Could you check a few things on this model? Use its own coordinates, in mm. Face numbers are marked on the shaded views. A direction names the side the tool comes from. Coordinates: 2 decimals unless noted, no trailing zeros. Order: outer loops, then holes, each group sorted by start corner. A loop starts at its lowest first (then second) coordinate and runs counter-clockwise, first axis right, second up. Notation, with made-up numbers: (63.25, -21.5) - (113.25, -21.5) arc R26 cw to (113.25, -3.5) - close; hole circle Ø7 at (11, -20). An arc over 180 degrees is marked (long way). One line per item, written item: value. Start each with the question number.
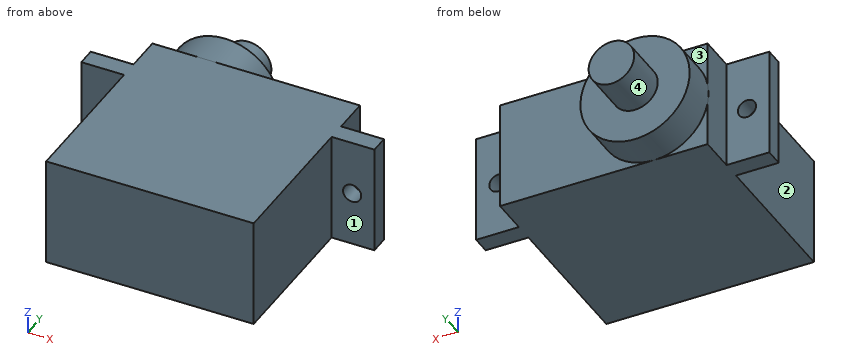
from build123d import *

# Parameters (mm, degrees)
SKETCH1_W           = 22.8
SKETCH1_H           = 12
BOSS_EXTRUDE1_DEPTH = 22.5
SKETCH2_W           = 12
SKETCH2_H           = 2
BOSS_EXTRUDE2_DEPTH = 4.7
SKETCH3_R           = 6
BOSS_EXTRUDE3_DEPTH = 4
SKETCH4_R           = 2.5
BOSS_EXTRUDE4_DEPTH = 5
SKETCH5_R           = 1
CUT_EXTRUDE1_DEPTH  = 5


with BuildPart() as part:
    # Sketch1 → Boss-Extrude1 (new body)
    with BuildSketch(Plane(origin=(0, 0, 0), x_dir=(1, 0, 0), z_dir=(0, 1, 0))):
        Rectangle(SKETCH1_W, SKETCH1_H)
    extrude(amount=BOSS_EXTRUDE1_DEPTH)

    # Sketch2 → Boss-Extrude2 (add)
    with BuildSketch(Plane(origin=(11.4, 0, 0), x_dir=(0, 0, -1), z_dir=(1, 0, 0))):
        with Locations((0, 17.5)):
            Rectangle(SKETCH2_W, SKETCH2_H)
    boss_extrude2 = extrude(amount=BOSS_EXTRUDE2_DEPTH)

    # Mirror1: Boss-Extrude2 across plane
    add(boss_extrude2.mirror(Plane(origin=(0, 0, 0), x_dir=(0, 0, 1), z_dir=(1, 0, 0))))

    # Sketch3 → Boss-Extrude3 (add)
    with BuildSketch(Plane(origin=(0, 22.5, 0), x_dir=(1, 0, 0), z_dir=(0, 1, 0))):
        with Locations(Location((-5.5, 0, 0), (0, 0, 270))):
            Circle(SKETCH3_R)
    extrude(amount=BOSS_EXTRUDE3_DEPTH)

    # Sketch4 → Boss-Extrude4 (add)
    with BuildSketch(Plane(origin=(0, 26.5, 0), x_dir=(1, 0, 0), z_dir=(0, 1, 0))):
        with Locations(Location((-5.5, 0, 0), (0, 0, 270))):
            Circle(SKETCH4_R)
    extrude(amount=BOSS_EXTRUDE4_DEPTH)

    # Sketch5 → Cut-Extrude1 (cut)
    with BuildSketch(Plane(origin=(0, 18.5, 0), x_dir=(1, 0, 0), z_dir=(0, 1, 0))):
        with Locations(Location((13.65, 0, 0), (0, 0, 270))):
            Circle(SKETCH5_R)
    cut_extrude1 = extrude(amount=-CUT_EXTRUDE1_DEPTH, mode=Mode.SUBTRACT)

    # Mirror2: Cut-Extrude1 across plane
    add(cut_extrude1.mirror(Plane(origin=(0, 0, 0), x_dir=(0, 0, 1), z_dir=(1, 0, 0))), mode=Mode.SUBTRACT)


solid = part.part
Q1. I want a section at C-C on y = 18. Please give me the cut outline in (x, z), then the cut area to 3 significant figures.
Q2. I want a section at B-B on x = 13.65. Please give me the cut outline in (y, z).
Q3. I want a section at A-A on z = 0. Please give me the cut outline in (x, y), then the cut area to 3 significant figures.
Q4. Which directions (+Z, -Z, +X, -X, +Y, -Y) give clear straight access to the entire face, cutting with the end or side of a thin tool? Please do the marked faces 1, 2, 3 and 4.
Q5. If I drill on L1, parallel to Z at x = -13.65, y = 17.55; L2, parallel to X at y = 17.2, z = 0; L3, parallel to Y at x = 6.5, z = -3.5, over which ranges is the centre line in solid material (lowest first)?
Q6. I want a section at D-D on x = -2.5. Please give me the cut outline in (y, z), then the cut area to 3 significant figures.
Q7. I'm going to push flat-ended pins straight in: pin 1 (2.5 mm diameter, centred on x = 14.5, z = -1, fed in from -Y); pin 2 (1 mm diameter, centred on x = 9.5, z = -1, fed in from -Y); pin 3 (4 mm diameter, centred on x = -12, y = 26, fed in from +Z); pin 4 (2 mm diameter, centred on y = 20, z = -0.5, fed in from -X). Where does each tip first touch, or does it pass through?
Values follow:
1. outline: (-16.1, -6) - (16.1, -6) - (16.1, 6) - (-16.1, 6) - close; hole circle Ø2 at (-13.65, 0); hole circle Ø2 at (13.65, 0)
1. area: 380 mm^2
2. outline: (16.5, -6) - (18.5, -6) - (18.5, -1) - (16.5, -1) - close; (16.5, 1) - (18.5, 1) - (18.5, 6) - (16.5, 6) - close
3. outline: (-16.1, 16.5) - (-14.65, 16.5) - (-14.65, 18.5) - (-16.1, 18.5) - close; (-12.65, 16.5) - (-11.4, 16.5) - (-11.4, 0) - (11.4, 0) - (11.4, 16.5) - (12.65, 16.5) - (12.65, 18.5) - (11.4, 18.5) - (11.4, 22.5) - (0.5, 22.5) - (0.5, 26.5) - (-3, 26.5) - (-3, 31.5) - (-8, 31.5) - (-8, 26.5) - (-11.5, 26.5) - (-11.5, 22.5) - (-11.4, 22.5) - (-11.4, 18.5) - (-12.65, 18.5) - close; (14.65, 16.5) - (16.1, 16.5) - (16.1, 18.5) - (14.65, 18.5) - close
3. area: 597 mm^2
4. face 1: +Z, -Z, +X, -Y
4. face 2: +Z, -Z, -X, -Y
4. face 3: +Z, -X, +Y
4. face 4: +Y
5. L1: z = -6 to -1, 1 to 6
5. L2: x = -16.1 to -14.65, -12.65 to 12.65, 14.65 to 16.1
5. L3: y = 0 to 22.5
6. outline: (0, -6) - (22.5, -6) - (22.5, -5.2) - (26.5, -5.2) - (26.5, 5.2) - (22.5, 5.2) - (22.5, 6) - (0, 6) - close
6. area: 312 mm^2
7. pin 1: stops at y = 16.5
7. pin 2: stops at y = 0
7. pin 3: stops at z = 3.97
7. pin 4: stops at x = -11.4
